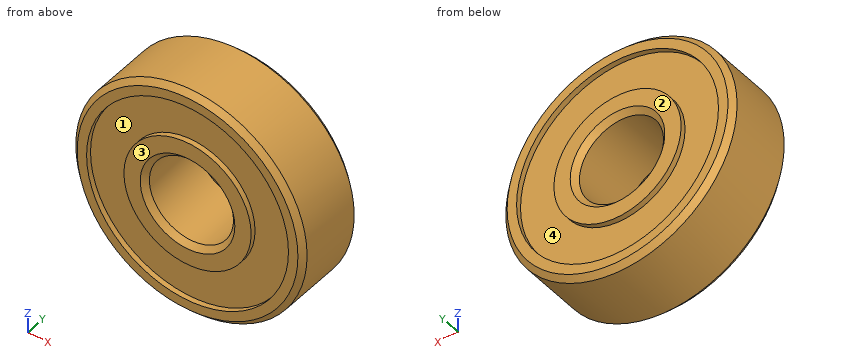
```python
from build123d import *

# Parameters (mm, degrees)
F0_R          = 11
F0_R_2        = 4
F1_DEPTH      = 6
F2_R          = 11
F2_R_2        = 9.6
F2_R_3        = 6.05
F2_R_4        = 4
F3_DEPTH      = 0.5
F3_DEPTH_BACK = 6.5
F4_SIZE       = 0.49999


# Not quite as in the source:
# - a fillet or chamfer is up to 0.001 mm smaller than in the source, because OpenCascade refuses the exact size


with BuildPart() as f1:
    # F0 (on Front) → F1 (new body)
    with BuildSketch(Plane.XZ):
        Circle(F0_R)
        Circle(F0_R_2, mode=Mode.SUBTRACT)
    extrude(amount=-F1_DEPTH)

    # F2 (on face) → F3 (join, two sides)
    with BuildSketch(Plane.XZ) as f3_sk:
        Circle(F2_R)
        Circle(F2_R_2, mode=Mode.SUBTRACT)
        Circle(F2_R_3)
        Circle(F2_R_4, mode=Mode.SUBTRACT)
    extrude(amount=F3_DEPTH)
    extrude(f3_sk.sketch, amount=-F3_DEPTH_BACK)

    # F4 (size 0.5 in the source; OpenCascade refuses exactly that, so slightly less here)
    f4_edges = [f1.edges().sort_by_distance(p)[0] for p in [
        (-11, -0.5, 0),
        (-4, -0.5, 0),
        (-11, 6.5, 0),
        (-4, 6.5, 0),
    ]]
    chamfer(f4_edges, length=F4_SIZE)


solid = f1.part
```
Input: part model. Units: mm. Frame: model coordinates. Face numbers are marked on the shaded views. A direction names the side the tool comes from. Round coordinates to 2 decimals unless told otherwise and drop trailing zeros. Loops run counter-clockwise (first coordinate to the right, second up) from the corner with the lowest first, then second, coordinate; pieces in that order, holes last. Notation, with made-up numbers: M 28.25,6.25 L 39.25,6.25 A14 ccw 39.25,32.25 Z; hole C -28.5,49 d4. An arc over 180 degrees is marked long. Answer in a Markdown table with one row per item. Add a question column.
1. Section C-C (y = 1.75). Output: boundary loops of the cut face in (x, z).
2. Ray query, probe 1 along Z at (x, y) = (0, 1.8); probe 2 along Y at (x, z) = (7.5, -4.25); probe 3 along Z at (x, y) = (-2, 6.25). Return the intervals inside material, ascending.
3. Mould query, pull axis Z, two halves, no side actions, for the marked faces 1 and 2. Classes: released by +Z, released by -Z, zero draft, split by the parting line, or undercut.
4. Contact query for flat-ended pins moving along their axis: pin 1 (3 mm diameter, centred on x = -6.5, y = 3, fed in from -Z); pin 2 (6.5 mm diameter, centred on x = 0, z = 0, fed in from -Y); pin 3 (1 mm diameter, centred on x = 5, y = 3.5, fed in from +Z); pin 4 (1 mm diameter, centred on y = 3.5, z = -8.5, fed in from +X). Output: stop coordinate, or through.
5. Set-up query: the marked faces 3 and 4. Return all of +Z, -Z, +X, -X, +Y, -Y with unobstructed straight access to the full face (end or side cutting, diameter ignored); none if empty.
Values follow:
| question | item | result |
|---|---|---|
| 1 | outline | C 0,0 d22; hole C 0,0 d8 |
| 2 | probe 1 | -11 to -4, 4 to 11 |
| 2 | probe 2 | 0 to 6 |
| 2 | probe 3 | -10.56 to -9.39, -5.71 to -3.75, 3.75 to 5.71, 9.39 to 10.56 |
| 3 | face 1 | undercut |
| 3 | face 2 | zero draft |
| 4 | pin 1 | z = -9.8 |
| 4 | pin 2 | through |
| 4 | pin 3 | z = 10.04 |
| 4 | pin 4 | x = 7.55 |
| 5 | face 3 | +Z, -Z, +X, -X, -Y |
| 5 | face 4 | +Y |
